For this review, take the finished solid that the model builds, in its own axes (mm). Face numbers are marked on the shaded views. Coordinates: 2 decimals unless noted, no trailing zeros. Write each loop counter-clockwise with the first axis right and the second up, starting at its lowest first coordinate (ties: lowest second). Pieces come first, ordered by that corner, then holes. Notation, with made-up numbers: M 5.5,52 L 39.5,52 A26 ccw 39.5,66 Z; hole C 34,43.5 d2. An arc over 180 degrees is marked long. Return JSON: item names as keys, results as strings.
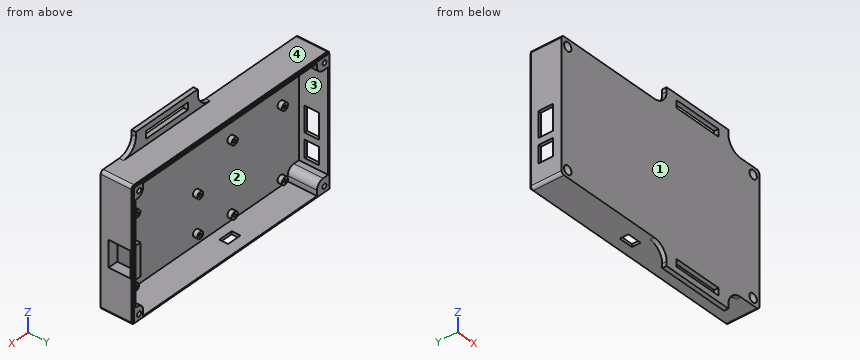
```python
from build123d import *

# Parameters (mm, degrees)
SKETCH1_W           = 160
SKETCH1_H           = 90
BOSS_EXTRUDE1_DEPTH = 22.2
SHELL1_T            = -2
SKETCH2_W           = 9.051657133
SKETCH2_H           = 7.429819316
SKETCH2_W_2         = 6.377912523
SKETCH2_H_2         = 8.717812211
BOSS_EXTRUDE2_DEPTH = 20.2
SKETCH5_W           = 160
SKETCH5_H           = 90
SKETCH5_W_2         = 157.8
SKETCH5_H_2         = 87.8
CUT_EXTRUDE2_DEPTH  = 1
SKETCH6_R           = 1.6
CUT_EXTRUDE3_DEPTH  = 25
SKETCH13_R          = 3
CUT_EXTRUDE8_DEPTH  = 15
SKETCH14_W          = 50
SKETCH14_H          = 3
BOSS_EXTRUDE4_DEPTH = 13
SKETCH15_W          = 34
SKETCH15_H          = 5
CUT_EXTRUDE9_DEPTH  = 10
SKETCH16_W          = 50
SKETCH16_H          = 3
BOSS_EXTRUDE5_DEPTH = 13
SKETCH17_W          = 34
SKETCH17_H          = 5
CUT_EXTRUDE10_DEPTH = 10
SKETCH22_W          = 12
SKETCH22_H          = 10
SKETCH22_W_2        = 17.5
CUT_EXTRUDE15_DEPTH = 10
SKETCH23_W          = 10
SKETCH23_H          = 6
CUT_EXTRUDE16_DEPTH = 10
FILLET1_R           = 10
FILLET4_R           = 5
FILLET9_R           = 2
SKETCH26_R          = 2.5
SKETCH26_R_2        = 2.4
BOSS_EXTRUDE7_DEPTH = 3
SKETCH27_R          = 1
CUT_EXTRUDE17_DEPTH = 2
SKETCH28_W          = 22
SKETCH28_H          = 19.5
BOSS_EXTRUDE8_DEPTH = 5
SKETCH29_W          = 18
SKETCH29_H          = 15
CUT_EXTRUDE18_DEPTH = 17


with BuildPart() as part:
    # Sketch1 → Boss-Extrude1 (new body)
    with BuildSketch(Plane(origin=(0, 0, 0), x_dir=(1, 0, 0), z_dir=(0, 1, 0))):
        with Locations((80, 45)):
            Rectangle(SKETCH1_W, SKETCH1_H)
    extrude(amount=BOSS_EXTRUDE1_DEPTH)

    # Shell1
    shell1_openings = [part.faces().sort_by_distance(p)[0] for p in [
        (80, 22.2, -45),
    ]]
    offset(amount=SHELL1_T, openings=shell1_openings, kind=Kind.INTERSECTION)

    # Sketch2 → Boss-Extrude2 (add)
    with BuildSketch(Plane(origin=(0, 2, 0), x_dir=(1, 0, 0), z_dir=(0, 1, 0))):
        with Locations((6.525828567, 5.714909658)):
            Rectangle(SKETCH2_W, SKETCH2_H)
        with Locations((154.811043739, 83.641093895)):
            Rectangle(SKETCH2_W_2, SKETCH2_H_2)
        with Locations((154.811043739, 5.714909658)):
            Rectangle(SKETCH2_W_2, SKETCH2_H)
        with Locations((6.525828567, 83.641093895)):
            Rectangle(SKETCH2_W, SKETCH2_H_2)
    extrude(amount=BOSS_EXTRUDE2_DEPTH)

    # Sketch5 → Cut-Extrude2 (cut)
    with BuildSketch(Plane(origin=(0, 22.2, 0), x_dir=(1, 0, 0), z_dir=(0, 1, 0))):
        with Locations((80, 45)):
            Rectangle(SKETCH5_W, SKETCH5_H)
        with Locations((80, 45)):
            Rectangle(SKETCH5_W_2, SKETCH5_H_2, mode=Mode.SUBTRACT)
    extrude(amount=-CUT_EXTRUDE2_DEPTH, mode=Mode.SUBTRACT)

    # Sketch6 → Cut-Extrude3 (cut)
    with BuildSketch(Plane(origin=(0, 22.2, 0), x_dir=(1, 0, 0), z_dir=(0, 1, 0))):
        with Locations(Location((155, 85, 0), (0, 0, 270))):
            Circle(SKETCH6_R)
        with Locations(Location((155, 5, 0), (0, 0, 270))):
            Circle(SKETCH6_R)
        with Locations(Location((5, 85, 0), (0, 0, 270))):
            Circle(SKETCH6_R)
        with Locations(Location((5, 5, 0), (0, 0, 270))):
            Circle(SKETCH6_R)
    extrude(amount=-CUT_EXTRUDE3_DEPTH, mode=Mode.SUBTRACT)

    # Sketch13 → Cut-Extrude8 (cut)
    with BuildSketch(Plane.XZ):
        with Locations(Location((155, -5, 0), (0, 0, 270))):
            Circle(SKETCH13_R)
        with Locations(Location((155, -85, 0), (0, 0, 270))):
            Circle(SKETCH13_R)
        with Locations(Location((5, -5, 0), (0, 0, 270))):
            Circle(SKETCH13_R)
        with Locations(Location((5, -85, 0), (0, 0, 270))):
            Circle(SKETCH13_R)
    extrude(amount=-CUT_EXTRUDE8_DEPTH, mode=Mode.SUBTRACT)

    # Sketch14 → Boss-Extrude4 (add)
    with BuildSketch(Plane.XY):
        with Locations((110, 1.5)):
            Rectangle(SKETCH14_W, SKETCH14_H)
    extrude(amount=BOSS_EXTRUDE4_DEPTH)

    # Sketch15 → Cut-Extrude9 (cut)
    with BuildSketch(Plane(origin=(0, 0, 0), x_dir=(-1, 0, 0), z_dir=(0, -1, 0))):
        with Locations((-110, -6.5)):
            Rectangle(SKETCH15_W, SKETCH15_H)
    extrude(amount=-CUT_EXTRUDE9_DEPTH, mode=Mode.SUBTRACT)

    # Sketch16 → Boss-Extrude5 (add)
    with BuildSketch(Plane(origin=(0, 0, -90), x_dir=(-1, 0, 0), z_dir=(0, 0, -1))):
        with Locations((-110, 1.5)):
            Rectangle(SKETCH16_W, SKETCH16_H)
    extrude(amount=BOSS_EXTRUDE5_DEPTH)

    # Sketch17 → Cut-Extrude10 (cut)
    with BuildSketch(Plane(origin=(0, 0, 0), x_dir=(-1, 0, 0), z_dir=(0, -1, 0))):
        with Locations((-110, 96.5)):
            Rectangle(SKETCH17_W, SKETCH17_H)
    extrude(amount=-CUT_EXTRUDE10_DEPTH, mode=Mode.SUBTRACT)

    # Sketch22 → Cut-Extrude15 (cut)
    with BuildSketch(Plane.ZY):
        with Locations((-70, 11)):
            Rectangle(SKETCH22_W, SKETCH22_H)
        with Locations((-50.75, 11)):
            Rectangle(SKETCH22_W_2, SKETCH22_H)
    extrude(amount=-CUT_EXTRUDE15_DEPTH, mode=Mode.SUBTRACT)

    # Sketch23 → Cut-Extrude16 (cut)
    with BuildSketch(Plane(origin=(0, 0, -90), x_dir=(-1, 0, 0), z_dir=(0, 0, -1))):
        with Locations((-69, 11.5)):
            Rectangle(SKETCH23_W, SKETCH23_H)
    extrude(amount=-CUT_EXTRUDE16_DEPTH, mode=Mode.SUBTRACT)

    # Fillet1
    fillet1_edges = [part.edges().sort_by_distance(p)[0] for p in [
        (135, 1.5, 0),
        (85, 1.5, 0),
        (135, 1.5, -90),
        (85, 1.5, -90),
    ]]
    fillet(fillet1_edges, radius=FILLET1_R)

    # Fillet4
    fillet4_edges = [part.edges().sort_by_distance(p)[0] for p in [
        (11.051657133, 12.1, -9.429819316),
        (151.622087477, 12.1, -79.282187789),
        (11.051657133, 12.1, -79.282187789),
        (151.622087477, 12.1, -9.429819316),
    ]]
    fillet(fillet4_edges, radius=FILLET4_R)

    # Fillet9
    fillet9_edges = [part.edges().sort_by_distance(p)[0] for p in [
        (0, 10.6, -90),
        (160, 10.6, -90),
        (160, 10.6, 0),
        (0, 10.6, 0),
    ]]
    fillet(fillet9_edges, radius=FILLET9_R)

    # Sketch26 → Boss-Extrude7 (add)
    with BuildSketch(Plane(origin=(0, 2, 0), x_dir=(1, 0, 0), z_dir=(0, 1, 0))):
        with Locations(Location((16.75, 83.2, 0), (0, 0, 90))):
            Circle(SKETCH26_R)
        with Locations(Location((16.75, 35, 0), (0, 0, 90))):
            Circle(SKETCH26_R)
        with Locations(Location((57.4, 35, 0), (0, 0, 90))):
            Circle(SKETCH26_R)
        with Locations(Location((57.4, 83.2, 0), (0, 0, 90))):
            Circle(SKETCH26_R)
        with Locations(Location((137.122087477, 85.5, 0), (0, 0, 90))):
            Circle(SKETCH26_R_2)
        with Locations(Location((136.122087477, 38.5, 0), (0, 0, 90))):
            Circle(SKETCH26_R_2)
        with Locations(Location((85.322087477, 54.478431373, 0), (0, 0, 90))):
            Circle(SKETCH26_R_2)
        with Locations(Location((85.322087477, 80.4, 0), (0, 0, 90))):
            Circle(SKETCH26_R_2)
    extrude(amount=BOSS_EXTRUDE7_DEPTH)

    # Sketch27 → Cut-Extrude17 (cut)
    with BuildSketch(Plane(origin=(0, 5, 0), x_dir=(1, 0, 0), z_dir=(0, 1, 0))):
        with Locations(Location((57.4, 83.2, 0), (0, 0, 270))):
            Circle(SKETCH27_R)
        with Locations(Location((57.4, 35, 0), (0, 0, 270))):
            Circle(SKETCH27_R)
        with Locations(Location((16.75, 35, 0), (0, 0, 270))):
            Circle(SKETCH27_R)
        with Locations(Location((16.75, 83.2, 0), (0, 0, 270))):
            Circle(SKETCH27_R)
        with Locations(Location((136.122087477, 38.5, 0), (0, 0, 270))):
            Circle(SKETCH27_R)
        with Locations(Location((137.122087477, 85.5, 0), (0, 0, 270))):
            Circle(SKETCH27_R)
        with Locations(Location((85.322087477, 80.4, 0), (0, 0, 270))):
            Circle(SKETCH27_R)
        with Locations(Location((85.322087477, 54.478431373, 0), (0, 0, 270))):
            Circle(SKETCH27_R)
    extrude(amount=-CUT_EXTRUDE17_DEPTH, mode=Mode.SUBTRACT)

    # Sketch28 → Boss-Extrude8 (add)
    with BuildSketch(Plane.ZY.offset(-158)):
        with Locations((-51, 11.75)):
            Rectangle(SKETCH28_W, SKETCH28_H)
    extrude(amount=BOSS_EXTRUDE8_DEPTH)

    # Sketch29 → Cut-Extrude18 (cut)
    with BuildSketch(Plane.ZY.offset(-153)):
        with Locations((-51, 13)):
            Rectangle(SKETCH29_W, SKETCH29_H)
    extrude(amount=-CUT_EXTRUDE18_DEPTH, mode=Mode.SUBTRACT)


solid = part.part
```
1. We need section C-C (z = -15.5). State the section outline as (x, y) points, plus the area to 3 significant figures.
Checks:
{"outline": "M 0,0 L 160,0 L 160,21.2 L 158.9,21.2 L 158.9,22.2 L 158,22.2 L 158,2 L 2,2 L 2,22.2 L 1.1,22.2 L 1.1,21.2 L 0,21.2 Z", "area": "399 mm2"}
2. We need section A-A (z = -66.5). State the section outline as (x, y) points.
Checks:
{"outline": "M 0,0 L 160,0 L 160,21.2 L 158.9,21.2 L 158.9,22.2 L 158,22.2 L 158,2 L 2,2 L 2,6 L 0,6 Z; M 0,16 L 2,16 L 2,22.2 L 1.1,22.2 L 1.1,21.2 L 0,21.2 Z"}
3. We need section D-D (x = 53). State the section outline as (y, z) points.
Checks:
{"outline": "M 0,-90 L 21.2,-90 L 21.2,-88.9 L 22.2,-88.9 L 22.2,-88 L 2,-88 L 2,-2 L 22.2,-2 L 22.2,-1.1 L 21.2,-1.1 L 21.2,0 L 0,0 Z"}
4. Wall thickness on L1, parallel to X at y = 18.25, z = -5; L2, parallel to X at y = 18, z = -85; L3, parallel to X at y = 3.8, z = -35: over which ranges is each line inside the solid? List them lowest first. Write a range as from..to.
Checks:
{"L1": "0..3.4, 6.6..11.02, 151.65..153.4, 156.6..160", "L2": "0..3.4, 6.6..11.05, 151.62..153.4, 156.6..160", "L3": "0..2, 14.25..15.75, 17.75..19.25, 54.9..56.4, 58.4..59.9, 158..160"}
5. Clearance check with flat-ended pins moving along their axes: pin 1 Ø7.5 at (x, y) = (156.5, 11) entering from -Z; pin 2 Ø1 at (x, y) = (57.5, 5.5) entering from +Z; pin 3 Ø1.5 at (y, z) = (2, 6.5) entering from +X. State where each tip first meets the part, or that it passes through.
Checks:
{"pin 1": "z = -90", "pin 2": "z = 0", "pin 3": "x = 135.95"}
6. We need section B-B (x = 107.5). State the section outline as (y, z) points.
Checks:
{"outline": "M 0,-103 L 3,-103 L 3,-99 L 0,-99 Z; M 0,-94 L 3,-94 L 3,-90 L 21.2,-90 L 21.2,-88.9 L 22.2,-88.9 L 22.2,-88 L 2,-88 L 2,-2 L 22.2,-2 L 22.2,-1.1 L 21.2,-1.1 L 21.2,0 L 3,0 L 3,4 L 0,4 Z; M 0,9 L 3,9 L 3,13 L 0,13 Z"}
7. Draft analysis for pull direction Z (two halves, no side actions). For the marked faces 1, 2, 3 and 4, state which applies: +Z half, -Z half, draft (parallel to the pull), parting line (faces both ways), or undercut.
Checks:
{"face 1": "draft", "face 2": "undercut", "face 3": "undercut", "face 4": "+Z half"}
